Work out the finished part from the listing and answer in its coordinate system (mm). Give positions to 0.01 mm unless a question says otherwise; leave off trailing zeros. Order: outer loops, then holes, each group sorted by start corner. A loop starts at its lowest first (then second) coordinate and runs counter-clockwise, first axis right, second up.
```python
from build123d import *

# Parameters (mm, degrees)
BOSS_EXTRUDE2_OUTLINE_W = 330.2
BOSS_EXTRUDE2_OUTLINE_H = 190.5
BOSS_EXTRUDE2_DEPTH     = 3
CUT_EXTRUDE1_DEPTH      = 554.733952504


# Read off the part's stored shape, not the designer's step: Boss-Extrude2
with BuildPart() as part:
    # Boss-Extrude2 outline → Boss-Extrude2 (new body)
    with BuildSketch(Plane.XY):
        with Locations((-165.1, 349.25)):
            Rectangle(BOSS_EXTRUDE2_OUTLINE_W, BOSS_EXTRUDE2_OUTLINE_H)
        with BuildLine():
            add(Edge.make_bspline(
                [(-305.942171993, 328.501522762), (-306.170255378, 328.324665909), (-306.614042299, 327.954986533), (-307.512202671, 327.084665698), (-309.028565354, 325.224006494), (-310.814681605, 321.397067185), (-310.908770444, 315.937871104), (-309.331820466, 311.311401642), (-307.336526947, 308.049254205), (-304.674018188, 305.304468379), (-300.585989718, 302.625100143), (-295.275340887, 301.356761249), (-291.124175679, 302.133615904), (-288.944522893, 303.138863231), (-287.877956893, 303.791999802), (-287.175136962, 304.298621856), (-286.509456581, 304.853140919), (-285.611296208, 305.723461755), (-284.094933526, 307.584120959), (-282.308817275, 311.411060268), (-282.214728435, 316.870256349), (-283.791678414, 321.496725811), (-285.786971933, 324.758873247), (-288.449480692, 327.503659074), (-292.537509162, 330.18302731), (-297.848157993, 331.451366204), (-301.999323201, 330.674511549), (-304.178975987, 329.669264222), (-305.245541986, 329.01612765), (-305.714088607, 328.678379615), (-305.942171993, 328.501522762)],
                knots=[0, 0, 0, 0, 0.015625, 0.03125, 0.0625, 0.125, 0.1875, 0.21875, 0.25, 0.28125, 0.3125, 0.375, 0.4375, 0.46875, 0.484375, 0.5, 0.515625, 0.53125, 0.5625, 0.625, 0.6875, 0.71875, 0.75, 0.78125, 0.8125, 0.875, 0.9375, 0.96875, 0.984375, 1, 1, 1, 1], degree=3))
        make_face(mode=Mode.SUBTRACT)
        with BuildLine():
            add(Edge.make_bspline(
                [(-180.068905291, 353.920439433), (-180.085422965, 353.618309147), (-180.081950788, 353.012052683), (-179.905256871, 351.701966023), (-179.071932531, 349.235984489), (-176.547678646, 346.101494923), (-171.788832257, 343.101891305), (-167.066920591, 341.126264084), (-161.345782684, 339.656260684), (-155.018201929, 338.900335341), (-148.645925657, 338.961950616), (-142.798632236, 339.799499783), (-137.889488846, 341.248590487), (-132.832001497, 343.711528272), (-129.981083909, 346.552153454), (-128.883895778, 348.912592521), (-128.565435113, 350.195608733), (-128.461120803, 351.099005754), (-128.466329068, 352.008390451), (-128.643022986, 353.31847711), (-129.476347326, 355.784458645), (-132.000601211, 358.918948211), (-136.7594476, 361.918551828), (-141.481359266, 363.89417905), (-147.202497173, 365.36418245), (-153.530077928, 366.120107793), (-159.9023542, 366.058492517), (-165.74964762, 365.220943351), (-170.658791011, 363.771852646), (-175.71627836, 361.308914861), (-178.567195948, 358.468289679), (-179.664384078, 356.107850612), (-179.982844744, 354.8248344), (-180.052387617, 354.22256972), (-180.068905291, 353.920439433)],
                knots=[0, 0, 0, 0, 0.015625, 0.03125, 0.0625, 0.125, 0.15625, 0.1875, 0.21875, 0.25, 0.28125, 0.3125, 0.34375, 0.375, 0.4375, 0.46875, 0.484375, 0.5, 0.515625, 0.53125, 0.5625, 0.625, 0.65625, 0.6875, 0.71875, 0.75, 0.78125, 0.8125, 0.84375, 0.875, 0.9375, 0.96875, 0.984375, 1, 1, 1, 1], degree=3))
        make_face(mode=Mode.SUBTRACT)
        with BuildLine():
            add(Edge.make_bspline(
                [(-29.09461346, 384.409392838), (-29.375319528, 384.349132794), (-29.932845744, 384.210511135), (-31.115639474, 383.827797032), (-33.287380866, 382.853955405), (-36.5808932, 380.334793707), (-39.113343797, 375.767453995), (-39.778124595, 371.238575823), (-39.453462961, 367.698185468), (-38.296430811, 364.336482677), (-35.831427961, 360.479484886), (-31.647527324, 357.353965166), (-27.610258166, 356.408525111), (-25.230170518, 356.411838769), (-23.994513151, 356.548301078), (-23.146566065, 356.701928853), (-22.310276741, 356.909861342), (-21.127483011, 357.292575445), (-18.955741619, 358.266417073), (-15.662229285, 360.78557877), (-13.129778688, 365.352918482), (-12.46499789, 369.881796654), (-12.789659524, 373.42218701), (-13.946691674, 376.7838898), (-16.411694524, 380.640887591), (-20.595595161, 383.766407311), (-24.632864319, 384.711847366), (-27.012951967, 384.708533708), (-28.248609334, 384.572071399), (-28.813907391, 384.469652882), (-29.09461346, 384.409392838)],
                knots=[0, 0, 0, 0, 0.015625, 0.03125, 0.0625, 0.125, 0.1875, 0.21875, 0.25, 0.28125, 0.3125, 0.375, 0.4375, 0.46875, 0.484375, 0.5, 0.515625, 0.53125, 0.5625, 0.625, 0.6875, 0.71875, 0.75, 0.78125, 0.8125, 0.875, 0.9375, 0.96875, 0.984375, 1, 1, 1, 1], degree=3))
        make_face(mode=Mode.SUBTRACT)
    extrude(amount=BOSS_EXTRUDE2_DEPTH)

    # Sketch9 → Cut-Extrude1 (cut, through all)
    with BuildSketch(Plane(origin=(0, 0, 0), x_dir=(-1, 0, 0), z_dir=(0, 0, -1))):
        Polygon((330.2, 444.5), (0, 444.5), (0, 389.89), (25.851104386, 389.89), (25.851104386, 344.17), (95.701104386, 344.17), (95.701104386, 374.65), (152.287972712, 374.65), (152.287972712, 326.39), (205.910863718, 326.39), (205.910863718, 337.82), (294.810863718, 337.82), (294.810863718, 254), (330.2, 254), align=None)
    extrude(amount=-CUT_EXTRUDE1_DEPTH, mode=Mode.SUBTRACT)


solid = part.part
```
1. Straight lines are drawn through the part: probe 1 along X at (y, z) = (352, 1.7); probe 2 along Y at (x, z) = (-194, 1.1); probe 3 along X at (y, z) = (334, 2.8). For each, find the intervals that lie inside material, in ascending order.
Findings below:
probe 1: x = -128.49 to -95.7, -25.85 to 0
probe 2: y = 254 to 326.39
probe 3: x = -294.81 to -205.91, -152.29 to 0
2. The part is cut by section B-B (x = -221). Write down the section's boundary in (y, z).
Findings below:
outline: (254, 0) - (337.82, 0) - (337.82, 3) - (254, 3) - close
3. The part is cut by section A-A (x = -68). Write down the section's boundary in (y, z), then the cut area to 3 significant figures.
Findings below:
outline: (254, 0) - (344.17, 0) - (344.17, 3) - (254, 3) - close
area: 271 mm2
4. Given P1, Ø0.9, axis at x = -170, z = 1.5, coming from the +Y side; P2, Ø1.5, axis at y = 368.5, z = 1.5, coming from the -X side; P3, Ø0.9, axis at x = -126.5, z = 2, coming from the +Y side, each flat-ended and moving along its own axis, determine where each tip first touches the part or whether it passes through.
Findings below:
P1: stops at y = 326.39
P2: stops at x = -152.29
P3: stops at y = 374.65
